Check sheet for the modelled part. Datum: model origin and axes. Units: mm. Face numbers are marked on the shaded views. Give positions to 0.01 mm unless a question says otherwise; leave off trailing zeros. Loops run counter-clockwise (first coordinate to the right, second up) from the corner with the lowest first, then second, coordinate; pieces in that order, holes last. Notation, with made-up numbers: M 65.25,43 L 99.25,43 A25 cw 99.25,60 Z; hole C 32,71.25 d3. An arc over 180 degrees is marked long. Write each question's results on one line, items separated by ' | '. Start each with the question number.
1. Sectioned sample at C-C on x = 0. Record the cut outline in (y, z), and give its area (3 significant figures).
2. Sectioned sample at A-A on z = 0. Record the cut outline in (x, y).
3. Draft check along Z on the marked faces 1, 2 and 3. Enter one of: pulls with the +Z half, pulls with the -Z half, needs draft (parallel to the pull), parting line crosses it, or undercut.
4. Go/stop test with flat-tipped pins: pin 1 (0.8 mm diameter, centred on x = 37.5, y = 24, fed in from -Z); pin 2 (3 mm diameter, centred on y = 23.5, z = 38, fed in from -X); pin 3 (3 mm diameter, centred on x = -40, y = 23, fed in from -Z). Record where each tip stops, or that it passes through.
5. Sectioned sample at D-D on x = -20. Record the cut outline in (y, z).
6. Sectioned sample at B-B on y = 13. Give the number of separate pieces and of enclosed holes in the cut face, and give its area (3 significant figures).
7. Material ranges on line 1 along X through (y, z) = (3.5, 1.5); line 2 along Z through (x, y) = (20, 14.25); line 3 along Y through (x, z) = (-24, 15), recorded low to high.
```python
from build123d import *
from build123d.topology import SkipClean

# Parameters (mm, degrees)
SKETCH1_R           = 53.75
SKETCH1_R_2         = 51.25
BOSS_EXTRUDE1_DEPTH = 25
BOSS_EXTRUDE2_START = 2.5
SKETCH6_R           = 53.75
BOSS_EXTRUDE2_DEPTH = 2.5
SKETCH8_R           = 4.5
SKETCH8_R_2         = 2
BOSS_EXTRUDE3_DEPTH = 25
BOSS_EXTRUDE4_START = -2.5
BOSS_EXTRUDE4_DEPTH = 2.5


with BuildPart() as part:
    # Sketch1 → Boss-Extrude1 (new body)
    with BuildSketch(Plane(origin=(0, 0, 0), x_dir=(1, 0, 0), z_dir=(0, 1, 0))):
        with Locations(Location((0, 0, 0), (0, 0, 270))):
            Circle(SKETCH1_R)
        with Locations(Location((0, 0, 0), (0, 0, 270))):
            Circle(SKETCH1_R_2, mode=Mode.SUBTRACT)
    extrude(amount=BOSS_EXTRUDE1_DEPTH)

    # Sketch6 → Boss-Extrude2 (add)
    with BuildSketch(Plane.XZ.offset(BOSS_EXTRUDE2_START)):
        with Locations(Location((0, 0, 0), (0, 0, 270))):
            Circle(SKETCH6_R)
    extrude(amount=-BOSS_EXTRUDE2_DEPTH)

    # Sketch8 → Boss-Extrude3 (add)
    # profile 1 of 4: a face of its own
    with BuildSketch(Plane(origin=(0, 0, 0), x_dir=(1, 0, 0), z_dir=(0, 1, 0))):
        with Locations(Location((-20, 20, 0), (0, 0, 90))):
            Circle(SKETCH8_R)
        with Locations(Location((-20, 20, 0), (0, 0, 270))):
            Circle(SKETCH8_R_2, mode=Mode.SUBTRACT)
    # profile 2 of 4: a face of its own
    with BuildSketch(Plane(origin=(0, 0, 0), x_dir=(1, 0, 0), z_dir=(0, 1, 0))):
        with Locations(Location((20, 20, 0), (0, 0, 90))):
            Circle(SKETCH8_R)
        with Locations(Location((20, 20, 0), (0, 0, 270))):
            Circle(SKETCH8_R_2, mode=Mode.SUBTRACT)
    # profile 3 of 4: a face of its own
    with BuildSketch(Plane(origin=(0, 0, 0), x_dir=(1, 0, 0), z_dir=(0, 1, 0))):
        with Locations(Location((20, -20, 0), (0, 0, 90))):
            Circle(SKETCH8_R)
        with Locations(Location((20, -20, 0), (0, 0, 270))):
            Circle(SKETCH8_R_2, mode=Mode.SUBTRACT)
    # profile 4 of 4: a face of its own
    with BuildSketch(Plane(origin=(0, 0, 0), x_dir=(1, 0, 0), z_dir=(0, 1, 0))):
        with Locations(Location((-20, -20, 0), (0, 0, 90))):
            Circle(SKETCH8_R)
        with Locations(Location((-20, -20, 0), (0, 0, 270))):
            Circle(SKETCH8_R_2, mode=Mode.SUBTRACT)
    extrude(amount=BOSS_EXTRUDE3_DEPTH)

    # Sketch12 → Boss-Extrude4 (add)
    with SkipClean():  # the faces are left unmerged after this step: merging them gives an invalid solid
        with BuildSketch(Plane(origin=(0, 25, 0), x_dir=(1, 0, 0), z_dir=(0, 1, 0)).offset(BOSS_EXTRUDE4_START)):
            with BuildLine():
                Line((-18.75, 18.4387505), (-18.75, -18.4387505))
                ThreePointArc((-18.75, -18.4387505), (-20, -18), (-21.25, -18.4387505))
                Line((-21.25, -18.4387505), (-21.25, 18.4387505))
                ThreePointArc((-21.25, 18.4387505), (-20, 18), (-18.75, 18.4387505))
            make_face()
            with BuildLine():
                Line((18.4387505, 21.25), (-18.4387505, 21.25))
                ThreePointArc((-18.4387505, 21.25), (-18, 20), (-18.4387505, 18.75))
                Line((-18.4387505, 18.75), (18.4387505, 18.75))
                ThreePointArc((18.4387505, 18.75), (18, 20), (18.4387505, 21.25))
            make_face()
            with BuildLine():
                Line((21.25, 18.4387505), (21.25, -18.4387505))
                ThreePointArc((21.25, -18.4387505), (20, -18), (18.75, -18.4387505))
                Line((18.75, -18.4387505), (18.75, 18.4387505))
                ThreePointArc((18.75, 18.4387505), (20, 18), (21.25, 18.4387505))
            make_face()
            with BuildLine():
                Line((18.4387505, -21.25), (-18.4387505, -21.25))
                ThreePointArc((-18.4387505, -21.25), (-18, -20), (-18.4387505, -18.75))
                Line((-18.4387505, -18.75), (18.4387505, -18.75))
                ThreePointArc((18.4387505, -18.75), (18, -20), (18.4387505, -21.25))
            make_face()
            with BuildLine():
                Line((-21.5612495, 21.25), (-49.371044145, 21.25))
                ThreePointArc((-49.371044145, 21.25), (-49.887986714, 20.006281055), (-50.373604199, 18.75))
                Line((-50.373604199, 18.75), (-21.5612495, 18.75))
                ThreePointArc((-21.5612495, 18.75), (-22, 20), (-21.5612495, 21.25))
            make_face()
            with BuildLine():
                Line((-21.25, 21.5612495), (-21.25, 49.371044145))
                ThreePointArc((-21.25, 49.371044145), (-20.006281055, 49.887986714), (-18.75, 50.373604199))
                Line((-18.75, 50.373604199), (-18.75, 21.5612495))
                ThreePointArc((-18.75, 21.5612495), (-20, 22), (-21.25, 21.5612495))
            make_face()
            with BuildLine():
                Line((18.75, 21.5612495), (18.75, 50.373604199))
                ThreePointArc((18.75, 50.373604199), (20.006281055, 49.887986714), (21.25, 49.371044145))
                Line((21.25, 49.371044145), (21.25, 21.5612495))
                ThreePointArc((21.25, 21.5612495), (20, 22), (18.75, 21.5612495))
            make_face()
            with BuildLine():
                Line((21.5612495, 21.25), (49.371044145, 21.25))
                ThreePointArc((49.371044145, 21.25), (49.887986714, 20.006281055), (50.373604199, 18.75))
                Line((50.373604199, 18.75), (21.5612495, 18.75))
                ThreePointArc((21.5612495, 18.75), (22, 20), (21.5612495, 21.25))
            make_face()
            with BuildLine():
                Line((18.75, -21.5612495), (18.75, -50.373604199))
                ThreePointArc((18.75, -50.373604199), (20.006281055, -49.887986714), (21.25, -49.371044145))
                Line((21.25, -49.371044145), (21.25, -21.5612495))
                ThreePointArc((21.25, -21.5612495), (20, -22), (18.75, -21.5612495))
            make_face()
            with BuildLine():
                Line((21.5612495, -21.25), (49.371044145, -21.25))
                ThreePointArc((49.371044145, -21.25), (49.887986714, -20.006281055), (50.373604199, -18.75))
                Line((50.373604199, -18.75), (21.5612495, -18.75))
                ThreePointArc((21.5612495, -18.75), (22, -20), (21.5612495, -21.25))
            make_face()
            with BuildLine():
                Line((-18.75, -21.5612495), (-18.75, -50.373604199))
                ThreePointArc((-18.75, -50.373604199), (-20.006281055, -49.887986714), (-21.25, -49.371044145))
                Line((-21.25, -49.371044145), (-21.25, -21.5612495))
                ThreePointArc((-21.25, -21.5612495), (-20, -22), (-18.75, -21.5612495))
            make_face()
            with BuildLine():
                Line((-21.5612495, -21.25), (-49.371044145, -21.25))
                ThreePointArc((-49.371044145, -21.25), (-49.887986714, -20.006281055), (-50.373604199, -18.75))
                Line((-50.373604199, -18.75), (-21.5612495, -18.75))
                ThreePointArc((-21.5612495, -18.75), (-22, -20), (-21.5612495, -21.25))
            make_face()
        extrude(amount=BOSS_EXTRUDE4_DEPTH)


solid = part.part
```
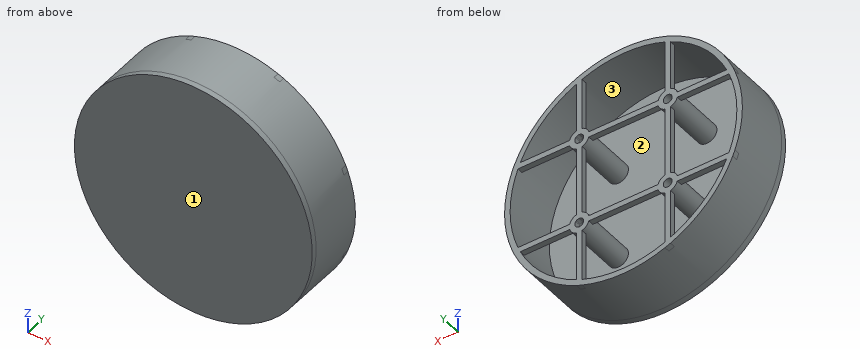
Output values:
1) outline: M -2.5,-53.75 L 25,-53.75 L 25,-51.25 L 0,-51.25 L 0,51.25 L 25,51.25 L 25,53.75 L -2.5,53.75 Z; M 22.5,-21.25 L 25,-21.25 L 25,-18.75 L 22.5,-18.75 Z; M 22.5,18.75 L 25,18.75 L 25,21.25 L 22.5,21.25 Z | area: 406 mm2
2) outline: M -53.75,-2.5 L 53.75,-2.5 L 53.75,25 L 51.25,25 L 51.25,0 L -51.25,0 L -51.25,25 L -53.75,25 Z; M -21.25,22.5 L -18.75,22.5 L -18.75,25 L -21.25,25 Z; M 18.75,22.5 L 21.25,22.5 L 21.25,25 L 18.75,25 Z
3) face 1: needs draft | face 2: undercut | face 3: undercut
4) pin 1: z = -38.89 | pin 2: x = -39.46 | pin 3: z = -37.51
5) outline: M -2.5,-49.89 L 25,-49.89 L 25,-22 L 0,-22 L 0,-18 L 25,-18 L 25,18 L 0,18 L 0,22 L 25,22 L 25,49.89 L -2.5,49.89 Z; hole M 0,-47.19 L 22.5,-47.19 L 22.5,-24.5 L 0,-24.5 Z; hole M 0,-15.5 L 22.5,-15.5 L 22.5,15.5 L 0,15.5 Z; hole M 0,24.5 L 22.5,24.5 L 22.5,47.19 L 0,47.19 Z
6) separate pieces: 5 | enclosed holes: 5 | area: 1,030 mm2
7) line 1: -53.73 to -51.23, 51.23 to 53.73 | line 2: -49.89 to -47.19, -24.5 to -22, -18 to -15.5, 15.5 to 18, 22 to 24.5, 47.19 to 49.89 | line 3: -2.5 to 0
